Design review of the part shown in the three views and the two pictorial views. Dimensions are in mm from the part's minimum x, y and z. A direction names the side the tool comes from. Coordinates: 2 decimals unless noted, no trailing zeros. Loops run counter-clockwise (first coordinate to the right, second up) from the corner with the lowest first, then second, coordinate; pieces in that order, holes last. Notation, with made-up numbers: (41, 88) - (58, 88) arc R34 cw to (58, 123) - close; hole circle Ø1 at (23, -0.75). An arc over 180 degrees is marked (long way). One line per question, with ' | ' between items.
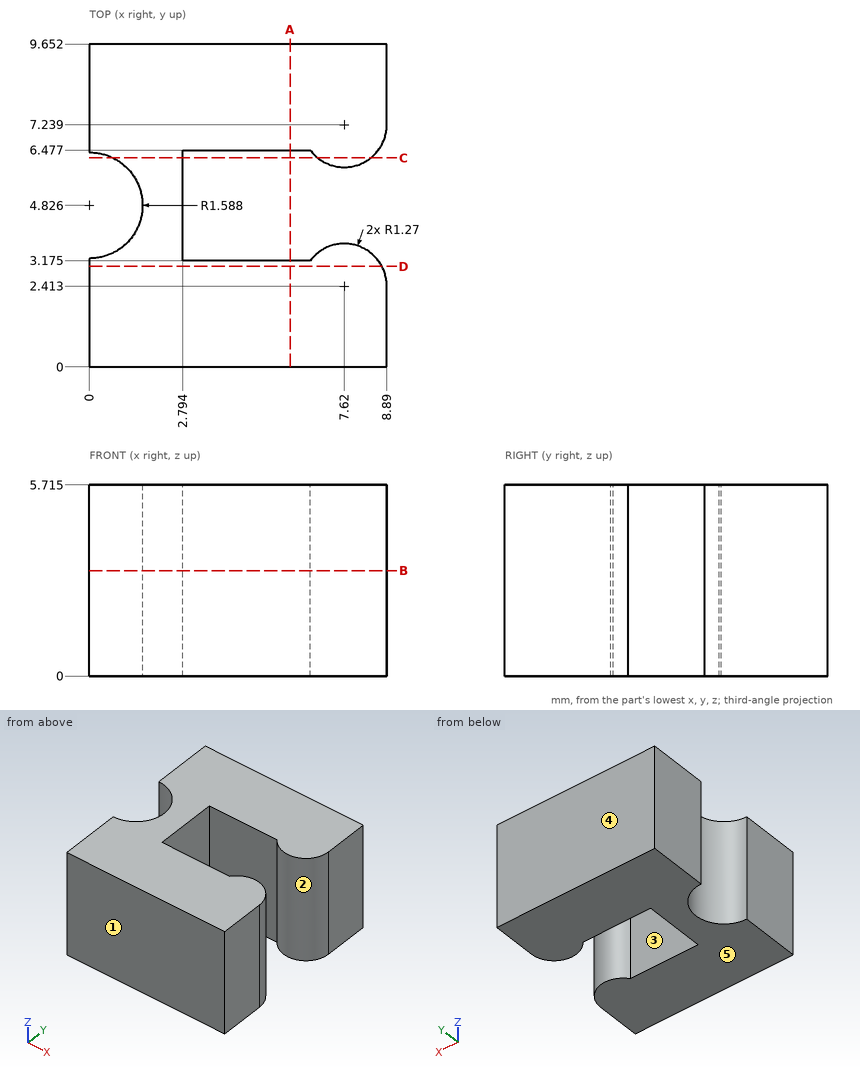
Q1. Take a section at A-A (x = 6). Give the boundary of the cut face in (y, z) (1 decimal).
Returned:
outline: (0, 0) - (3.2, 0) - (3.2, 5.7) - (0, 5.7) - close; (6.5, 0) - (9.7, 0) - (9.7, 5.7) - (6.5, 5.7) - close
Q2. Take a section at D-D (y = 3). Give the boundary of the cut face in (x, z) (1 decimal).
Returned:
outline: (0, 0) - (8.7, 0) - (8.7, 5.7) - (0, 5.7) - close
Q3. Tool access review of the marked faces 1 and 2: name each direction out of +Z, -Z, +X, -X, +Y, -Y from which nothing blocks a thin tool from reaching the whole face with its end or side.
Returned:
face 1: +Z, -Z, +X, -X, -Y | face 2: +Z, -Z
Q4. To check wall thickness, follow line 1 along Y through (x, z) = (6, 3.3) (1 decimal); line 2 along X through (y, z) = (2.5, 4.4); line 3 along Y through (x, z) = (7.25, 0.9) (1 decimal). State the ranges of each line that lie inside material, in increasing order.
Returned:
line 1: y = 0 to 3.2, 6.5 to 9.7 | line 2: x = 0 to 8.89 | line 3: y = 0 to 3.6, 6 to 9.7
Q5. Take a section at B-B (z = 3.15). Give the boundary of the cut face in (x, y) (1 decimal).
Returned:
outline: (0, 0) - (8.9, 0) - (8.9, 2.4) arc R1.3 ccw to (6.6, 3.2) - (2.8, 3.2) - (2.8, 6.5) - (6.6, 6.5) arc R1.3 ccw to (8.9, 7.2) - (8.9, 9.7) - (0, 9.7) - (0, 6.4) arc R1.6 cw to (0, 3.2) - close
Q6. Draft analysis for pull direction Y (two halves, no side actions). For the marked faces 3, 4 and 5, state which applies: +Y half, -Y half, draft (parallel to the pull), parting line (faces both ways), or undercut.
Returned:
face 3: undercut | face 4: +Y half | face 5: draft
Q7. For pin 1 (1.7 mm diameter, centred on y = 5.5, z = 2.5, fed in from +X) (1 decimal), flat-tipped, find the tip position at first contact; note if it passes through.
Returned:
pin 1: stops at x = 8.5
Q8. Take a section at C-C (y = 6.25). Give the boundary of the cut face in (x, z) (1 decimal).
Returned:
outline: (0.7, 0) - (2.8, 0) - (2.8, 5.7) - (0.7, 5.7) - close; (6.8, 0) - (8.4, 0) - (8.4, 5.7) - (6.8, 5.7) - close
